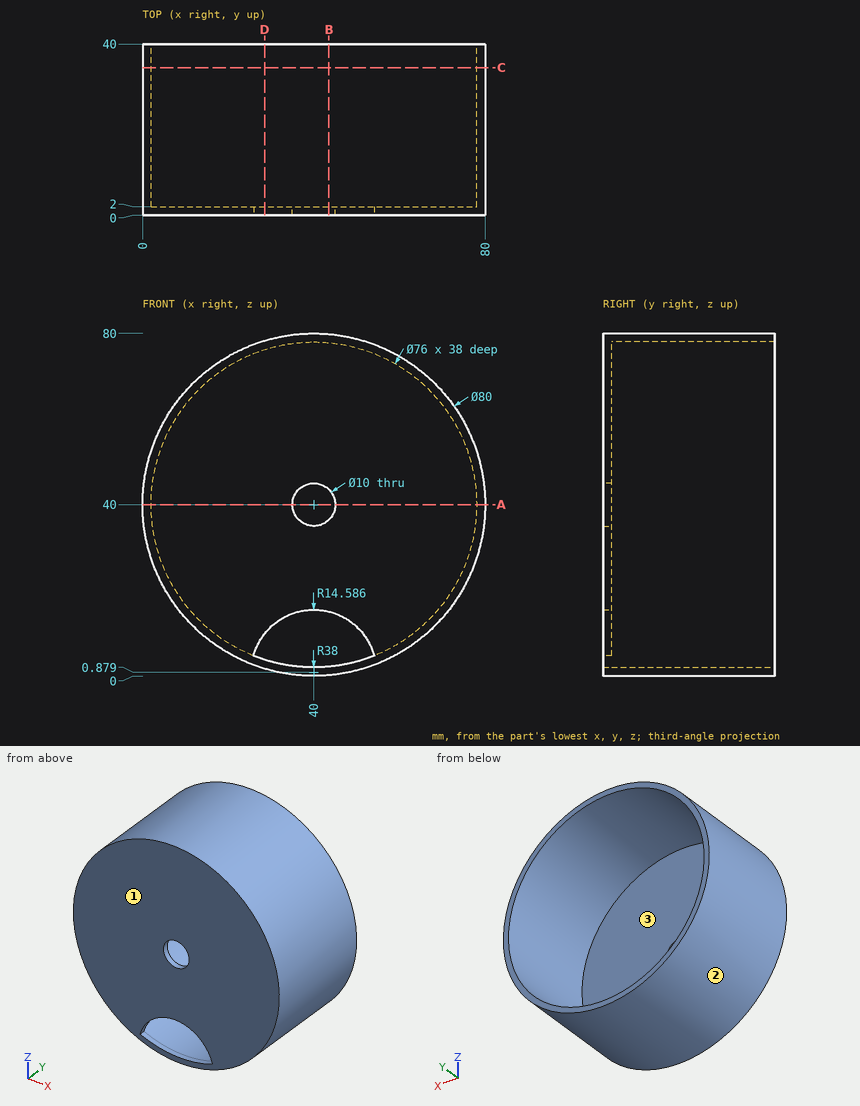
Drawing for the job (mm, zero at the part's lowest x, y, z). Round coordinates to 2 decimals unless told otherwise and drop trailing zeros. Order: outer loops, then holes, each group sorted by start corner. A loop starts at its lowest first (then second) coordinate and runs counter-clockwise, first axis right, second up. Notation, with made-up numbers: (28, 25) -> (60, 25) arc R27 cw to (60, 51) -> close; hole circle Ø1 at (24.5, 71.5). An arc over 180 degrees is marked (long way). Put each result on its own line as item: value.
Q1. Wall check: line 1 (X direction, y = 1.1, z = 40); line 2 (X direction, y = 14, z = 40); line 3 (Y direction, x = 44, z = 63.5). Give the ranges that are in metal, low to high. Write a range as [from, to].
From the geometry:
line 1: x = [0, 35], [45, 80]
line 2: x = [0, 2], [78, 80]
line 3: y = [0, 2]
Q2. Band-saw the part on A-A (z = 40). Give the cut face in (x, y), and give its area (3 significant figures).
From the geometry:
outline: (0, 0) -> (35, 0) -> (35, 2) -> (2, 2) -> (2, 40) -> (0, 40) -> close; (45, 0) -> (80, 0) -> (80, 40) -> (78, 40) -> (78, 2) -> (45, 2) -> close
area: 292 mm2
Q3. Pull direction X, two halves, no side cores. Call the marked faces 1, 2 and 3: pulls with the +X half, pulls with the -X half, needs draft (parallel to the pull), parting line crosses it, or undercut.
From the geometry:
face 1: needs draft
face 2: parting line crosses it
face 3: undercut
Q4. Band-saw the part on B-B (x = 43.5). Give the cut face in (y, z).
From the geometry:
outline: (0, 0.15) -> (40, 0.15) -> (40, 2.16) -> (0, 2.16) -> close; (0, 15.04) -> (2, 15.04) -> (2, 36.43) -> (0, 36.43) -> close; (0, 43.57) -> (2, 43.57) -> (2, 77.84) -> (40, 77.84) -> (40, 79.85) -> (0, 79.85) -> close
Q5. Band-saw the part on D-D (x = 28.5). Give the cut face in (y, z), and give its area (3 significant figures).
From the geometry:
outline: (0, 1.69) -> (40, 1.69) -> (40, 3.78) -> (0, 3.78) -> close; (0, 9.85) -> (2, 9.85) -> (2, 76.22) -> (40, 76.22) -> (40, 78.31) -> (0, 78.31) -> close
area: 300 mm2
Q6. Band-saw the part on C-C (y = 34.5). Give the cut face in (x, z), and give its area (3 significant figures).
From the geometry:
outline: circle Ø80 at (40, 40); hole circle Ø76 at (40, 40)
area: 490 mm2
Q7. Pin check, flat tips, straight feed: pin 1 Ø8 at (x, z) = (48.5, 10.5) entering from +Y; pin 2 Ø12 at (y, z) = (19, 29) entering from -X; pin 3 Ø3 at (y, z) = (24, 63) entering from +X. Stop position of each tip, or through.
From the geometry:
pin 1: stops at y = 2
pin 2: stops at x = 0.31
pin 3: stops at x = 73.73
